The listing builds one solid part. Answer for the finished solid, in the listing's coordinates (mm). A direction names the side the tool comes from. Round coordinates to 2 decimals unless told otherwise and drop trailing zeros. Write each loop counter-clockwise with the first axis right and the second up, starting at its lowest first coordinate (ties: lowest second). Pieces come first, ordered by that corner, then holes. Notation, with made-up numbers: M -6.5,85 L 32.5,85 A32 ccw 32.5,115 Z; hole C -24,62.25 d2. An arc over 180 degrees is marked long. Write each question's results on one line, items separated by ' | '.
from build123d import *

# Parameters (mm, degrees)
F0_W     = 75
F0_H     = 15
F1_DEPTH = 2
F2_W     = 69.8
F2_H     = 9.8
F3_DEPTH = 4
F4_R     = 5
F5_R     = 3
F6_R     = 5
F7_R     = 5
F8_R     = 3
F9_R     = 3
F10_R    = 5
F11_R    = 3


with BuildPart() as f1:
    # F0 (on Top) → F1 (new body)
    with BuildSketch(Plane.XY):
        with Locations((34.641778, -0.255361)):
            Rectangle(F0_W, F0_H)
    extrude(amount=F1_DEPTH)

    # F2 (on face) → F3 (join)
    with BuildSketch(Plane.XY.offset(2)):
        with Locations((34.641778, -0.255361)):
            Rectangle(F2_W, F2_H)
    extrude(amount=F3_DEPTH)

    # F4
    f4_edges = [f1.edges().sort_by_distance(p)[0] for p in [
        (-2.858222, -7.755361, 1),
    ]]
    fillet(f4_edges, radius=F4_R)

    # F5
    f5_edges = [f1.edges().sort_by_distance(p)[0] for p in [
        (-0.258222, -5.155361, 4),
    ]]
    fillet(f5_edges, radius=F5_R)

    # F6
    f6_edges = [f1.edges().sort_by_distance(p)[0] for p in [
        (72.141778, 7.244639, 1),
    ]]
    fillet(f6_edges, radius=F6_R)

    # F7
    f7_edges = [f1.edges().sort_by_distance(p)[0] for p in [
        (72.141778, -7.755361, 1),
    ]]
    fillet(f7_edges, radius=F7_R)

    # F8
    f8_edges = [f1.edges().sort_by_distance(p)[0] for p in [
        (69.541778, 4.644639, 4),
    ]]
    fillet(f8_edges, radius=F8_R)

    # F9
    f9_edges = [f1.edges().sort_by_distance(p)[0] for p in [
        (69.541778, -5.155361, 4),
    ]]
    fillet(f9_edges, radius=F9_R)

    # F10
    f10_edges = [f1.edges().sort_by_distance(p)[0] for p in [
        (-2.858222, 7.244639, 1),
    ]]
    fillet(f10_edges, radius=F10_R)

    # F11
    f11_edges = [f1.edges().sort_by_distance(p)[0] for p in [
        (-0.258222, 4.644639, 4),
    ]]
    fillet(f11_edges, radius=F11_R)


solid = f1.part
1) A tool of negligible diameter and unlimited length cuts with its end or side. For faces 1 (the face through (34, 4.645, 4)), 2 (the face through (34, -5.155, 4)), 3 (the face through (0.644, -4.3, 4.028)), from which of +Z, -Z, +X, -X, +Y, -Y can it reach the whole face along a straight path? Write none if from no direction.
Return value:
face 1: +Z, +X, -X, +Y | face 2: +Z, +X, -X, -Y | face 3: +Z, -X, -Y
2) Each of these flat-tipped pins is pushed along its axis until it touches: pin 1 (1.1 mm diameter, centred on y = -1, z = 3.5, fed in from -X); pin 2 (3 mm diameter, centred on y = 0, z = 4, fed in from +X); pin 3 (1.2 mm diameter, centred on x = 34.5, z = 4, fed in from +Y). Where does it stop, or does it pass through?
Return value:
pin 1: x = -0.26 | pin 2: x = 69.54 | pin 3: y = 4.64
3) Section C-C (y = 5.75) is taken. Determine the outline of the cut face in (x, z).
Return value:
outline: M -1.42,0 L 70.71,0 L 70.71,2 L -1.42,2 Z
4) Section B-B (z = 4.05) is taken. Determine the outline of the cut face in (x, y).
Return value:
outline: M -0.26,-2.16 A3 ccw 2.74,-5.16 L 66.54,-5.16 A3 ccw 69.54,-2.16 L 69.54,1.64 A3 ccw 66.54,4.64 L 2.74,4.64 A3 ccw -0.26,1.64 Z
5) Find the intervals of material crossed by line 1 (Y direction, x = 64.5, z = 5.1); line 2 (Z direction, x = 42.5, y = 5); line 3 (X direction, y = 0.5, z = 2.7), in increasing order.
Return value:
line 1: -5.16 to 4.64 | line 2: 0 to 2 | line 3: -0.26 to 69.54
6) Section A-A (x = 60) is taken. Determine the outline of the cut face in (y, z).
Return value:
outline: M -7.76,0 L 7.24,0 L 7.24,2 L 4.64,2 L 4.64,6 L -5.16,6 L -5.16,2 L -7.76,2 Z
